Could you check a few things on this model? Use its own coordinates, in mm. Face numbers are marked on the shaded views. A direction names the side the tool comes from. Give positions to 0.01 mm unless a question says otherwise; leave off trailing zeros. Order: outer loops, then holes, each group sorted by start corner. A loop starts at its lowest first (then second) coordinate and runs counter-clockwise, first axis right, second up. Notation, with made-up numbers: (37.25, 15.25) -> (87.25, 15.25) arc R19 ccw to (87.25, 40.25) -> close; hole circle Ø8 at (-2, 25). An arc over 180 degrees is marked (long way). Write each question's results on one line, items separated by ' | '.
```python
from build123d import *

# Parameters (mm, degrees)
F2_R     = 31.5
F3_DEPTH = 40


with BuildPart() as f1:
    # F0 (on Front) → F1 (revolve)
    with BuildSketch(Plane.XZ):
        with BuildLine():
            Line((-35, 0), (0, 0))
            Line((0, 0), (0, 272.395989))
            ThreePointArc((0, 272.395989), (-5.180591, 271.786704), (-10.090656, 270.025733))
            Line((-10.090656, 270.025733), (-71, 240))
            Line((-71, 240), (-71, 223.14471))
            Line((-71, 223.14471), (-50, 223.14471))
            Line((-50, 223.14471), (-50, 70.386211))
            Line((-50, 70.386211), (-35, 45))
            Line((-35, 45), (-35, 0))
        make_face()
    revolve(axis=Axis((0, 0, 137.5), (0, 0, -1)))

    # F2 (on face) → F3 (cut)
    with BuildSketch(Plane(origin=(0, 0, 0), x_dir=(1, 0, 0), z_dir=(0, 0, -1))):
        Circle(F2_R)
    extrude(amount=-F3_DEPTH, mode=Mode.SUBTRACT)


solid = f1.part
```
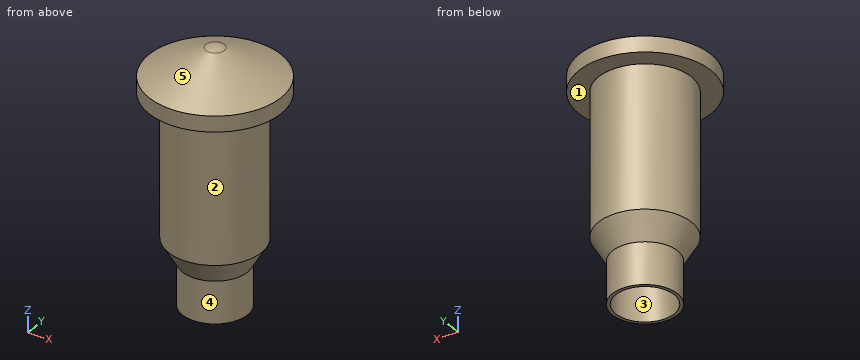
Q1. Thinking about a two-plate mould opening in Y: for the marked faces 1, 2 and 3, which applies, +Y half, -Y half, draft (parallel to the pull), parting line (faces both ways), or undercut?
Here are the results:
face 1: draft | face 2: parting line | face 3: undercut
Q2. Suppose I cut it at A-A on z = 176.5. Please give me the cut outline in (x, y), and give its area (3 significant figures).
Here are the results:
outline: circle Ø100 at (0, 0) | area: 7,850 mm²
Q3. I'm going to push flat-ended pins straight in: pin 1 Ø1 at (x, z) = (9.5, 177.5) entering from -Y; pin 2 Ø1 at (x, z) = (-21.5, 214) entering from +Y; pin 3 Ø6 at (x, y) = (56, 22.5) entering from -Z. Where does each tip first touch, or does it pass through?
Here are the results:
pin 1: stops at y = -49.18 | pin 2: stops at y = 45.38 | pin 3: stops at z = 223.14
Q4. For the marked faces 4 and 5, which set-ups out of +Z, -Z, +X, -X, +Y, -Y let a thin tool reach every point of the face, with its end or its side?
Here are the results:
face 4: -Z | face 5: +Z
Q5. I need wall thicknesses on line 1 along X through (y, z) = (-1.5, 12); line 2 along Y through (x, z) = (0, 23.5); line 3 along Y through (x, z) = (-4.5, 25.5). Which ranges of each line are inside material? Lowest first, please.
Here are the results:
line 1: x = -34.97 to -31.46, 31.46 to 34.97 | line 2: y = -35 to -31.5, 31.5 to 35 | line 3: y = -34.71 to -31.18, 31.18 to 34.71
